Geometry check sheet. Reference: the model listing, model coordinates, mm. A direction names the side the tool comes from. Coordinates: 2 decimals unless noted, no trailing zeros. Loops run counter-clockwise (first coordinate to the right, second up) from the corner with the lowest first, then second, coordinate; pieces in that order, holes last. Notation, with made-up numbers: (12, 41) - (62, 41) arc R16 ccw to (62, 54) - close; hole circle Ø1 at (11.5, 20.25). An arc over 180 degrees is marked (long way). One line per item, written item: value.
Autodesk Fusion 360 part; units mm, degrees
sketch "スケッチ1" plane through (0, 0, 0) normal (0, 0, 1) x (1, 0, 0)
  arc A0 (5, 11.5) -> (11.5, 5) centre (11.5, 11.5) ccw
  line L0 (0, 45) -> (0, 0)
  line L1 (45, 5) -> (11.5, 5)
  line L2 (0, 0) -> (45, 0)
  line L3 (45, 0) -> (45, 5)
  line L4 (5, 11.5) -> (5, 45)
  line L5 (5, 45) -> (0, 45)
extrude "押し出し1" add sketch "スケッチ1" along normal blind 100
(1) Cross-section at B-B on y = 26.5. Record the cut outline in (x, z).
Reply:
outline: (0, 0) - (5, 0) - (5, 100) - (0, 100) - close
(2) Access from +Z, -Z, +X, -X, +Y, -Y to the whole of each face (thin tool, end or side, straight path). Record for faces 1 (the face through (28, 5, 49)), 2 (the face through (0, 23, 49)).
Reply:
face 1: +Z, -Z, +X, +Y
face 2: +Z, -Z, -X, +Y, -Y
(3) Cross-section at A-A on z = 24.5. Record the cut outline in (x, y).
Reply:
outline: (0, 0) - (45, 0) - (45, 5) - (11.5, 5) arc R6.5 cw to (5, 11.5) - (5, 45) - (0, 45) - close
(4) Material ranges on probe 1 along Y at (x, z) = (18.5, 41); probe 2 along Y at (x, z) = (9, 84), recorded low to high. Write a range as from..to.
Reply:
probe 1: 0..5
probe 2: 0..5.5
(5) Go/stop test with flat-tipped pins: pin 1 Ø12 at (x, z) = (34.5, 46) entering from +Y; pin 2 Ø10 at (y, z) = (14.5, 81.5) entering from +X. Record where each tip stops, or that it passes through.
Reply:
pin 1: y = 5
pin 2: x = 5.32
